Autodesk Inventor part; units mm, degrees
ref_plane "YZ Plane" through (0, 0, 0) normal (1, 0, 0) x (0, 1, 0)
ref_plane "XZ Plane" through (0, 0, 0) normal (0, 1, 0) x (-1, 0, 0)
ref_plane "XY Plane" through (0, 0, 0) normal (0, 0, 1) x (1, 0, 0)
sketch "Sketch1" plane through (0, 0, 0) normal (0, 0, 1) x (1, 0, 0)
  line L0 (-57, -57.5) -> (57, 57.5) construction
  line L1 (-67.5, 67.5) -> (67.5, 67.5) construction
  line L2 (67.5, 67.5) -> (67.5, -67.5) construction
  line L3 (67.5, -67.5) -> (-67.5, -67.5) construction
  line L4 (-67.5, -67.5) -> (-67.5, 67.5) construction
  line L5 (-67.5, 67.5) -> (67.5, -67.5) construction
  line L6 (67.5, 67.5) -> (-67.5, -67.5) construction
  circle A0 centre (-37.5, 37.5) radius 4
  circle A1 centre (-37.5, -37.5) radius 4
  circle A2 centre (37.5, -37.5) radius 4
  circle A3 centre (37.5, 37.5) radius 4
  arc A4 (-48.5, 62.5) -> (-48.5, -62.5) centre (326.325, 0) ccw
  line L7 (0, 67.5) -> (0, -67.5) construction
  line L8 (67.5, -67.5) -> (67.5, 67.5) construction
  arc A5 (48.5, -62.5) -> (48.5, 62.5) centre (-326.325, 0) ccw
  arc A6 (48.5, 62.5) -> (-48.5, 62.5) centre (0, -110.8429) ccw
  line L9 (-67.5, 0) -> (53.675, 0) construction
  arc A7 (-48.5, -62.5) -> (48.5, -62.5) centre (0, 110.8429) ccw
  arc A8 (-30.7003, 46.1842) -> (-30.7003, -46.1842) centre (326.325, 0) ccw
  arc A9 (-30.7003, -46.1842) -> (30.7003, -46.1842) centre (0, 110.8429) ccw
  arc A10 (30.7003, -46.1842) -> (30.7003, 46.1842) centre (-326.325, 0) ccw
  arc A11 (30.7003, 46.1842) -> (-30.7003, 46.1842) centre (0, -110.8429) ccw
  arc A12 (-55.5322, 68.7683) -> (-55.5322, -68.7683) centre (326.325, 0) ccw
  arc A13 (-55.5322, -68.7683) -> (55.5322, -68.7683) centre (0, 110.8429) ccw
  arc A14 (55.5322, -68.7683) -> (55.5322, 68.7683) centre (-326.325, 0) ccw
  arc A15 (55.5322, 68.7683) -> (-55.5322, 68.7683) centre (0, -110.8429) ccw
  arc A16 (-57.2838, 70.3161) -> (-57.2838, -70.3161) centre (326.325, 0) ccw
  arc A17 (-57.2838, -70.3161) -> (57.2838, -70.3161) centre (0, 110.8429) ccw
  arc A18 (57.2838, -70.3161) -> (57.2838, 70.3161) centre (-326.325, 0) ccw
  arc A19 (57.2838, 70.3161) -> (-57.2838, 70.3161) centre (0, -110.8429) ccw
  line L10 (17.7854, 76.314) -> (17.0881, 68.3442)
  line L11 (38.478, 73.1774) -> (37.0881, 65.2948)
  line L12 (-17.7854, 76.314) -> (-17.0881, 68.3442)
  line L13 (-38.478, 73.1774) -> (-37.0881, 65.2948)
  line L14 (17.7854, -76.314) -> (17.0881, -68.3442)
  line L15 (38.478, -73.1774) -> (37.0881, -65.2948)
  line L16 (-38.478, -73.1774) -> (-37.0881, -65.2948)
  line L17 (-17.7854, -76.314) -> (-17.0881, -68.3442)
  point P0 (0, 0)
  point P1 (0, 0)
  point P2 (-53.675, 0)
  point P3 (0, 0)
  dimension "d3" = 135
  dimension "d4" = 135
  dimension "d5" = 8
  dimension "d9" = 360
  dimension "d29" = 75
  dimension "d30" = 125
  dimension "d31" = 97
  dimension "d32" = 180
  dimension "d33" = 380
  dimension "d34" = 20
  dimension "d36" = 8
  dimension "d37" = 2
  dimension "d38" = 5
  dimension "d39" = 20
  dimension "d41" = 5
extrude "Extrusion1" add sketch "Sketch1" along normal mid plane 220 contours L13 A15 L12 A6 | A7 L17 A13 L16 | L10 A15 L11 A6 | A7 L15 A13 L14 | A19 A18 A17 A16
fillet "Fillet2" radius 15 8 edges at (57.2838, 70.3161, 0) (-57.2838, 70.3161, 0) (-57.2838, -70.3161, 0) (57.2838, -70.3161, 0) (55.5322, -68.7683, 0) (-55.5322, -68.7683, 0) (-55.5322, 68.7683, 0) (55.5322, 68.7683, 0)
properties part number "lineaire as deel 2" material "Aluminum 6061"
Model file for the job. Use its own axes, mm. A direction names the side the tool comes from. Give positions to 0.01 mm unless a question says otherwise; leave off trailing zeros. Loops run counter-clockwise (first coordinate to the right, second up) from the corner with the lowest first, then second, coordinate; pieces in that order, holes last.
1) Flat gauge pins, fed straight in: pin 1 Ø1.5 at (x, z) = (-20, -71.5) entering from +Y; pin 2 Ø2 at (y, z) = (-36.5, 15.5) entering from +X; pin 3 Ø2 at (y, z) = (-13.5, 46.5) entering from +X. Where does each tip first touch, or does it go through?
2) Pull direction Y, two halves, no side cores. Call faces 3 (the cylindrical face through (0.677, -79.156, -1.54)), 4 (the cylindrical face through (61.674, 0.832, -1.54)), 5 (the cylindrical face through (-63.674, -0.855, -1.54)): +Y half, -Y half, draft (parallel to the pull), parting line (faces both ways), or undercut.
3) Wall check: line 1 (Y direction, x = 1.5, z = 21); line 2 (X direction, y = 42, z = 56.5); line 3 (X direction, y = -29, z = -45.5). Give the ranges that are in metal, low to high.
4) Saw through at A-A (x = -6). Write the cut outline in (y, z).
5) Tool access for faces 1 (the cylindrical face through (42.29, -72.34, -1.54)), 2 (the cylindrical face through (-0.677, 79.156, -1.54)): list every direction of +Z, -Z, +X, -X, +Y, -Y with a clear straight run to the whole face (end or side of a thin tool).
6) Saw through at B-B (y = -28). Write the cut outline in (x, z).
Answer block:
1. pin 1: stops at y = 78.18
1. pin 2: stops at x = 62.06
1. pin 3: stops at x = 63.47
2. face 3: -Y half
2. face 4: undercut
2. face 5: parting line
3. line 1: y = -79.15 to -77.15, 77.15 to 79.15
3. line 2: x = -61.41 to -59.4, 59.4 to 61.41
3. line 3: x = -62.6 to -60.59, 60.59 to 62.6
4. outline: (-79.06, -110) - (-77.06, -110) - (-77.06, 110) - (-79.06, 110) - close; (77.06, -110) - (79.06, -110) - (79.06, 110) - (77.06, 110) - close
5. face 1: +Z, -Z
5. face 2: +Z, -Z, +Y
6. outline: (-62.67, -110) - (-60.66, -110) - (-60.66, 110) - (-62.67, 110) - close; (60.66, -110) - (62.67, -110) - (62.67, 110) - (60.66, 110) - close
